Input: part model. Units: mm. Frame: model coordinates. Face numbers are marked on the shaded views. A direction names the side the tool comes from. Round coordinates to 2 decimals unless told otherwise and drop trailing zeros. Order: outer loops, then holes, each group sorted by start corner. A loop starts at its lowest first (then second) coordinate and runs counter-clockwise, first axis right, second up. Notation, with made-up numbers: (38, 74.5) - (58, 74.5) arc R25 ccw to (58, 101.5) - close; hole circle Ø8 at (-26.5, 43.25). An arc over 180 degrees is marked (long way). One line per item, written item: value. Start each with the question number.
from build123d import *

# Parameters (mm, degrees)
SKETCH1_R                                           = 28.575
SKETCH1_R_2                                         = 32.1437
BOSS_EXTRUDE1_DEPTH                                 = 25.4
CBORE_FOR_00_BINDING_HEAD_MACHINE_SCREW_D           = 10.16
CBORE_FOR_00_BINDING_HEAD_MACHINE_SCREW_CBORE_D     = 15.24
CBORE_FOR_00_BINDING_HEAD_MACHINE_SCREW_CBORE_DEPTH = 9.652
F_1_4_20_TAPPED_HOLE1_D                             = 5.1054
F_1_4_20_TAPPED_HOLE1_DEPTH                         = 17.516183098
F_1_4_20_TAPPED_HOLE1_TIP                           = 1.533816902
SKETCH5_R                                           = 77.7875
CUT_EXTRUDE1_DEPTH                                  = 6.35
F_5_16_18_TAPPED_HOLE1_D                            = 6.604
CIRPATTERN1_COUNT                                   = 6


with BuildPart() as part:
    # Sketch1 → Boss-Extrude1 (new body)
    with BuildSketch(Plane(origin=(0, 0, 0), x_dir=(1, 0, 0), z_dir=(0, 1, 0))):
        with BuildLine():
            Line((-95.25, 107.95), (-95.25, -107.95))
            ThreePointArc((-95.25, -107.95), (-89.670384182, -121.420384182), (-76.2, -127))
            Line((-76.2, -127), (107.95, -127))
            Line((107.95, -127), (250.077327963, -106.884827963))
            ThreePointArc((250.077327963, -106.884827963), (342.9, 0), (250.077327963, 106.884827963))
            Line((250.077327963, 106.884827963), (107.95, 127))
            Line((107.95, 127), (-76.2, 127))
            ThreePointArc((-76.2, 127), (-89.670384182, 121.420384182), (-95.25, 107.95))
        make_face()
        with Locations(Location((0, 0, 0), (0, 0, 270))):
            Circle(SKETCH1_R, mode=Mode.SUBTRACT)
        with Locations(Location((234.95, 0, 0), (0, 0, 270))):
            Circle(SKETCH1_R_2, mode=Mode.SUBTRACT)
    extrude(amount=BOSS_EXTRUDE1_DEPTH)

    # CBORE for #00 Binding Head Machine Screw1 (through all)
    with Locations(Plane(origin=(-76.2, 25.4, -107.95), x_dir=(0, 0, 1), z_dir=(0, 1, 0))):
        with Locations((0, 0), (215.9, 0), (0, 184.15), (215.9, 184.15)):
            CounterBoreHole(CBORE_FOR_00_BINDING_HEAD_MACHINE_SCREW_D / 2, CBORE_FOR_00_BINDING_HEAD_MACHINE_SCREW_CBORE_D / 2, CBORE_FOR_00_BINDING_HEAD_MACHINE_SCREW_CBORE_DEPTH)

    # 1/4-20 Tapped Hole1
    with Locations(Plane(origin=(-44.45, 25.4, -95.25), x_dir=(0, 0, 1), z_dir=(0, 1, 0))):
        with Locations((0, 0), (0, 88.9), (38.1, 88.9), (38.1, 0), (152.4, 0), (152.4, 88.9), (190.5, 88.9), (190.5, 0)):
            Hole(F_1_4_20_TAPPED_HOLE1_D / 2, depth=F_1_4_20_TAPPED_HOLE1_DEPTH)
            with Locations((0, 0, -(F_1_4_20_TAPPED_HOLE1_DEPTH + F_1_4_20_TAPPED_HOLE1_TIP / 2))):  # 118° drill point
                Cone(0, F_1_4_20_TAPPED_HOLE1_D / 2, F_1_4_20_TAPPED_HOLE1_TIP, mode=Mode.SUBTRACT)

    # Sketch5 → Cut-Extrude1 (cut)
    with BuildSketch(Plane(origin=(0, 25.4, 0), x_dir=(1, 0, 0), z_dir=(0, 1, 0))):
        with Locations(Location((234.95, 0, 0), (0, 0, 270))):
            Circle(SKETCH5_R)
    extrude(amount=-CUT_EXTRUDE1_DEPTH, mode=Mode.SUBTRACT)

    # 5/16-18 Tapped Hole1 (through all)
    with Locations(Plane(origin=(298.45, 19.05, 0), x_dir=(0, 0, 1), z_dir=(0, 1, 0))):
        with Locations((0, 0)):
            f_5_16_18_tapped_hole1 = Hole(F_5_16_18_TAPPED_HOLE1_D / 2)

    # CirPattern1: 5/16-18 Tapped Hole1 ×6 about axis
    cirpattern1_axis = Axis((234.95, 0, 0), (0, 1, 0))
    for i in range(1, CIRPATTERN1_COUNT):
        add(f_5_16_18_tapped_hole1.rotate(cirpattern1_axis, i * 360 / CIRPATTERN1_COUNT), mode=Mode.SUBTRACT)


solid = part.part
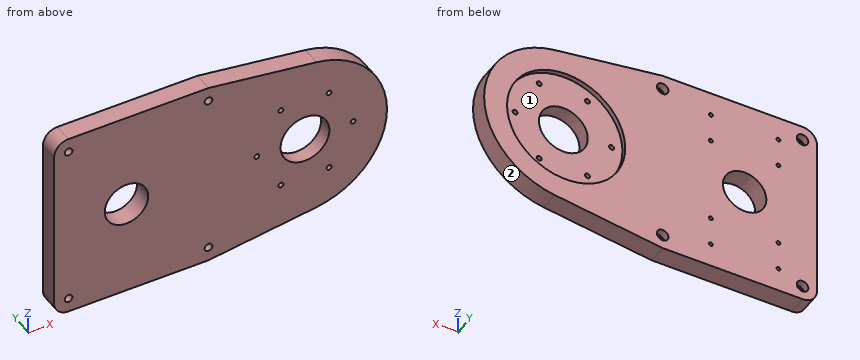
Item 1: First-contact query: pin 1 Ø4 at (x, z) = (-44.45, 95.25) entering from +Y; pin 2 Ø6 at (x, y) = (223.5, 8) entering from +Z; pin 3 Ø12 at (x, z) = (-20.5, -79.5) entering from -Y; pin 4 Ø13 at (x, z) = (-76.2, 107.95) entering from +Y. Flat tips, straight axial feed; report the tip coordinate or a pass-through.
Item 2: Section query D-D on x = 140. Return loops of the section in (y, z), and give its area (3 significant figures).
Item 3: Section query B-B on z = 67. Return loops of the section in (x, y).
Item 4: Section query C-C on x = 275.5. Return loops of the section in (y, z), and give its area (3 significant figures).
Item 5: Reachability of the marked faces 1 and 2 from +Z, -Z, +X, -X, +Y, -Y: full face, straight path, thin tool, end or side. Return the list, or none.
Item 6: Line query: L1, parallel to X at y = 11.5, z = 0 (3 decimals); L2, parallel to Z at x = -44.45, y = 21.5; L3, parallel to X at y = 18.75, z = 1.5. Output: solid intervals per line, ascending.
Item 7: Section query A-A on x = 19. Return loops of the section in (y, z).
Geometry results:
1. pin 1: stops at y = 7.55
1. pin 2: stops at z = 111.07
1. pin 3: stops at y = 0
1. pin 4: stops at y = 15.75
2. outline: (0, -122.46) - (25.4, -122.46) - (25.4, 122.46) - (0, 122.46) - close
2. area: 6,220 mm^2
3. outline: (-95.25, 0) - (319.59, 0) - (319.59, 25.4) - (274.47, 25.4) - (274.47, 19.05) - (195.43, 19.05) - (195.43, 25.4) - (-95.25, 25.4) - close
4. outline: (0, -100.04) - (25.4, -100.04) - (25.4, -66.38) - (19.05, -66.38) - (19.05, 66.38) - (25.4, 66.38) - (25.4, 100.04) - (0, 100.04) - close
4. area: 4,240 mm^2
5. face 1: +Y
5. face 2: +X, +Y, -Y
6. L1: x = -95.25 to -28.575, 28.575 to 168.148, 174.752 to 202.806, 267.094 to 295.148, 301.752 to 342.9
6. L2: z = -127 to -97.8, -92.7 to -59.7, -54.6 to 54.6, 59.7 to 92.7, 97.8 to 127
6. L3: x = -95.25 to -28.54, 28.54 to 168.51, 174.39 to 202.84, 267.06 to 295.51, 301.39 to 342.89
7. outline: (0, -127) - (25.4, -127) - (25.4, -21.34) - (0, -21.34) - close; (0, 21.34) - (25.4, 21.34) - (25.4, 127) - (0, 127) - close
